Check sheet for the modelled part. Datum: model origin and axes. Units: mm. A direction names the side the tool comes from. Round coordinates to 2 decimals unless told otherwise and drop trailing zeros. Write each loop counter-clockwise with the first axis right and the second up, starting at its lowest first coordinate (ties: lowest second). Pieces come first, ordered by that corner, then holes. Notation, with made-up numbers: (-3, 88) -> (50, 88) arc R24 ccw to (50, 114) -> close; hole circle Ø9 at (-24.75, 49.5). An arc over 180 degrees is marked (long way). One line per item, written item: value.
from build123d import *

# Parameters (mm, degrees)
SKETCH1_R           = 12.5
BOSS_EXTRUDE1_DEPTH = 51.8
SKETCH2_R           = 3.5
BOSS_EXTRUDE2_DEPTH = 2.5
SKETCH3_R           = 2
BOSS_EXTRUDE3_DEPTH = 10
SKETCH4_R           = 1.65
CUT_EXTRUDE1_DEPTH  = 5


with BuildPart() as part:
    # Sketch1 → Boss-Extrude1 (new body)
    with BuildSketch(Plane(origin=(0, 0, 0), x_dir=(1, 0, 0), z_dir=(0, 1, 0))):
        with Locations(Location((0, 0, 0), (0, 0, 90))):
            Circle(SKETCH1_R)
    extrude(amount=BOSS_EXTRUDE1_DEPTH)

    # Sketch2 → Boss-Extrude2 (add)
    with BuildSketch(Plane(origin=(0, 0, 0), x_dir=(-1, 0, 0), z_dir=(0, -1, 0))):
        with Locations(Location((0, 0, 0), (0, 0, 270))):
            Circle(SKETCH2_R)
    extrude(amount=BOSS_EXTRUDE2_DEPTH)

    # Sketch3 → Boss-Extrude3 (add)
    with BuildSketch(Plane(origin=(0, -2.5, 0), x_dir=(-1, 0, 0), z_dir=(0, -1, 0))):
        with Locations(Location((0, 0, 0), (0, 0, 90))):
            Circle(SKETCH3_R)
    extrude(amount=BOSS_EXTRUDE3_DEPTH)

    # Sketch4 → Cut-Extrude1 (cut)
    with BuildSketch(Plane(origin=(0, 0, 0), x_dir=(-1, 0, 0), z_dir=(0, -1, 0))):
        with Locations(Location((8.5, 0, 0), (0, 0, 90))):
            Circle(SKETCH4_R)
        with Locations(Location((-8.5, 0, 0), (0, 0, 90))):
            Circle(SKETCH4_R)
    extrude(amount=-CUT_EXTRUDE1_DEPTH, mode=Mode.SUBTRACT)


solid = part.part
Item 1: Sectioned sample at A-A on z = 0. Enter the section's corners in (x, y).
Answer:
outline: (-12.5, 0) -> (-10.15, 0) -> (-10.15, 5) -> (-6.85, 5) -> (-6.85, 0) -> (-3.5, 0) -> (-3.5, -2.5) -> (-2, -2.5) -> (-2, -12.5) -> (2, -12.5) -> (2, -2.5) -> (3.5, -2.5) -> (3.5, 0) -> (6.85, 0) -> (6.85, 5) -> (10.15, 5) -> (10.15, 0) -> (12.5, 0) -> (12.5, 51.8) -> (-12.5, 51.8) -> close
Item 2: Depth check by flat-ended pin: P1, Ø1, axis at x = 8, z = 1, coming from the -Y side; P2, Ø12, axis at x = -9.5, y = 32.5, coming from the -Z side; P3, Ø1, axis at x = 1, y = 9, coming from the +Z side. Enter the tip coordinate at first touch or a pass-through.
Answer:
P1: stops at y = 5
P2: stops at z = -12
P3: stops at z = 12.49
Item 3: Sectioned sample at C-C on x = 8.5. Enter the section's corners in (y, z), and give its area (3 significant figures).
Answer:
outline: (0, -9.17) -> (51.8, -9.17) -> (51.8, 9.17) -> (0, 9.17) -> (0, 1.65) -> (5, 1.65) -> (5, -1.65) -> (0, -1.65) -> close
area: 933 mm^2
Item 4: Sectioned sample at D-D on y = 32. Enter the section's corners in (x, z).
Answer:
outline: circle Ø25 at (0, 0)
Item 5: Sectioned sample at B-B on y = 2. Enter the section's corners in (x, z).
Answer:
outline: circle Ø25 at (0, 0); hole circle Ø3.3 at (-8.5, 0); hole circle Ø3.3 at (8.5, 0)
Item 6: Thickness scan on line 1 (X direction, y = 2.1, z = 0); line 2 (Y direction, x = -3, z = 7); line 3 (Y direction, x = -8, z = -1). Record the ranges inside material, lowest first.
Answer:
line 1: x = -12.5 to -10.15, -6.85 to 6.85, 10.15 to 12.5
line 2: y = 0 to 51.8
line 3: y = 5 to 51.8
Item 7: Mould release check, pull along X, two halves, no side actions. Record for faces 3 (the flat face through (0, 51.8, 0)), 4 (the cylindrical face through (-3.755, 25.537, -11.923)), 5 (the flat face through (-8, 5, 0)): pulls with the +X half, pulls with the -X half, needs draft (parallel to the pull), parting line crosses it, or undercut.
Answer:
face 3: needs draft
face 4: parting line crosses it
face 5: undercut
Item 8: Tool access check on faces 1 (the flat face through (2, -2.5, 2)), 2 (the flat face through (0, -12.5, 0)). Record the directions out of +Z, -Z, +X, -X, +Y, -Y that give a thin tool (end or side, any length) a straight path to the whole face; none if there is none.
Answer:
face 1: -Y
face 2: +Z, -Z, +X, -X, -Y
